Read the model definition and answer for the solid it produces. Units are mm, in the model's axes. Face numbers are marked on the shaded views. Give positions to 0.01 mm unless a question says otherwise; leave off trailing zeros. Loops run counter-clockwise (first coordinate to the right, second up) from the corner with the lowest first, then second, coordinate; pieces in that order, holes last. Notation, with made-up numbers: (-26, -37) - (29, -37) arc R23 cw to (29, 0) - close; hole circle Ø2 at (83, 16.5). An arc over 180 degrees is marked (long way). Write item = value, one per line.
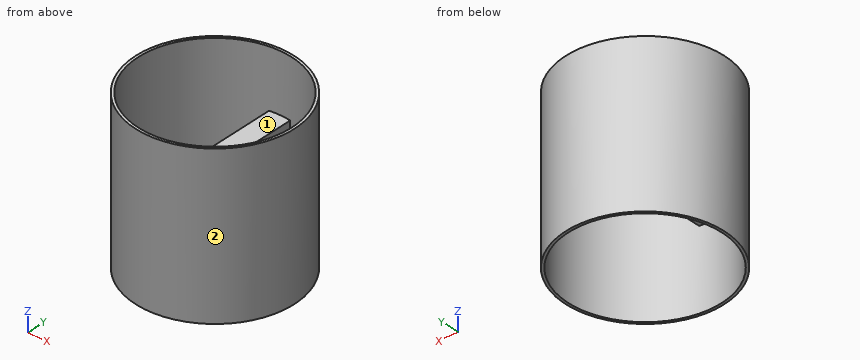
```python
from build123d import *

# Parameters (mm, degrees)
ESQUISSE1_W             = 8
ESQUISSE1_H             = 59
BOSS_EXTRU_1_DEPTH      = 60
ESQUISSE3_R             = 30
ESQUISSE3_R_2           = 29
BOSS_EXTRU_2_DEPTH      = 60
ESQUISSE4_R             = 29
ENL_V_MAT_EXTRU_3_DEPTH = 30
ENL_V_MAT_EXTRU_5_DEPTH = 1.5
ESQUISSE6_R             = 29
ENL_V_MAT_EXTRU_6_DEPTH = 22
ESQUISSE7_R             = 2
ENL_V_MAT_EXTRU_7_DEPTH = 6.5
ESQUISSE9_R             = 2
BOSS_EXTRU_4_DEPTH      = 6.5
ESQUISSE10_R            = 2
ENL_V_MAT_EXTRU_8_DEPTH = 3.7
ESQUISSE11_R            = 0.75
ENL_V_MAT_EXTRU_9_DEPTH = 3.7


with BuildPart() as part:
    # Esquisse1 → Boss.-Extru.1 (new body)
    with BuildSketch(Plane.XY):
        with Locations((4, 29.5)):
            Rectangle(ESQUISSE1_W, ESQUISSE1_H)
    extrude(amount=BOSS_EXTRU_1_DEPTH)

    # Esquisse3 → Boss.-Extru.2 (add)
    with BuildSketch(Plane(origin=(0, 0, 0), x_dir=(-1, 0, 0), z_dir=(0, 0, -1))):
        with Locations((-4, 29.5)):
            Circle(ESQUISSE3_R)
        with Locations((-4, 29.5)):
            Circle(ESQUISSE3_R_2, mode=Mode.SUBTRACT)
    extrude(amount=-BOSS_EXTRU_2_DEPTH)

    # Esquisse4 → Enlèv. mat.-Extru.3 (cut)
    with BuildSketch(Plane(origin=(0, 0, 0), x_dir=(-1, 0, 0), z_dir=(0, 0, -1))):
        with Locations((-4, 29.5)):
            Circle(ESQUISSE4_R)
    extrude(amount=-ENL_V_MAT_EXTRU_3_DEPTH, mode=Mode.SUBTRACT)

    # Esquisse5 → Enlèv. mat.-Extru.5 (cut)
    with BuildSketch(Plane(origin=(0, 0, 30), x_dir=(-1, 0, 0), z_dir=(0, 0, -1))):
        with BuildLine():
            Line((-6, 43), (-6.967257844, 29.9420191))
            ThreePointArc((-6.967257844, 29.9420191), (-7, 29.5), (-6.967257844, 29.0579809))
            Line((-6.967257844, 29.0579809), (-6, 16))
            ThreePointArc((-6, 16), (-4, 14), (-2, 16))
            Line((-2, 16), (-1.032742156, 29.0579809))
            ThreePointArc((-1.032742156, 29.0579809), (-1, 29.5), (-1.032742156, 29.9420191))
            Line((-1.032742156, 29.9420191), (-2, 43))
            ThreePointArc((-2, 43), (-4, 45), (-6, 43))
        make_face()
    extrude(amount=-ENL_V_MAT_EXTRU_5_DEPTH, mode=Mode.SUBTRACT)

    # Esquisse6 → Enlèv. mat.-Extru.6 (cut)
    with BuildSketch(Plane.XY.offset(60)):
        with Locations((4, 29.5)):
            Circle(ESQUISSE6_R)
    extrude(amount=-ENL_V_MAT_EXTRU_6_DEPTH, mode=Mode.SUBTRACT)

    # Esquisse7 → Enlèv. mat.-Extru.7 (cut)
    with BuildSketch(Plane(origin=(0, 0, 31.5), x_dir=(-1, 0, 0), z_dir=(0, 0, -1))):
        with Locations((-4, 29.5)):
            Circle(ESQUISSE7_R)
    extrude(amount=-ENL_V_MAT_EXTRU_7_DEPTH, mode=Mode.SUBTRACT)

    # Esquisse9 → Boss.-Extru.4 (add)
    with BuildSketch(Plane.XY.offset(38)):
        with Locations((4, 29.5)):
            Circle(ESQUISSE9_R)
    extrude(amount=-BOSS_EXTRU_4_DEPTH)

    # Esquisse10 → Enlèv. mat.-Extru.8 (cut)
    with BuildSketch(Plane.XY.offset(38)):
        with Locations((4, 29.5)):
            Circle(ESQUISSE10_R)
    extrude(amount=-ENL_V_MAT_EXTRU_8_DEPTH, mode=Mode.SUBTRACT)

    # Esquisse11 → Enlèv. mat.-Extru.9 (cut)
    with BuildSketch(Plane.XY.offset(34.3)):
        with Locations((4, 29.5)):
            Circle(ESQUISSE11_R)
    extrude(amount=-ENL_V_MAT_EXTRU_9_DEPTH, mode=Mode.SUBTRACT)


solid = part.part
```
1) A cutting plane is placed at C-C on z = 46. Determine the outline of the cut face in (x, y).
Output:
outline = circle Ø60 at (4, 29.5); hole circle Ø58 at (4, 29.5)
2) Find the intervals of material crossed by probe 1 along Y at (x, z) = (4, 36.05); probe 2 along Y at (x, z) = (4.5, 57.5); probe 3 along X at (y, z) = (43, 36), in increasing order.
Output:
probe_1 = -0.5 to 27.5, 31.5 to 59.5
probe_2 = -0.5 to 0.5, 58.5 to 59.5
probe_3 = -22.79 to -21.67, 0 to 8, 29.67 to 30.79
3) A cutting plane is placed at D-D on x = 17.5. Determine the outline of the cut face in (y, z).
Output:
outline = (2.71, 0) - (3.83, 0) - (3.83, 60) - (2.71, 60) - close; (55.17, 0) - (56.29, 0) - (56.29, 60) - (55.17, 60) - close
4) Each of these flat-tipped pins is pushed along its axis until it touches: P1, Ø4.5, axis at x = 4.5, y = 28.5, coming from the +Z side; P2, Ø1.5, axis at x = 9.5, y = 20, coming from the +Z side; P3, Ø4, axis at y = 41.5, z = 33.5, coming from the +X side; P4, Ø10, axis at x = -18.5, z = 12.5, coming from the -Y side. Where does it stop, or does it pass through?
Output:
P1 = 38
P2 = through
P3 = 32.28
P4 = 5.13
5) A cutting plane is placed at A-A on y = 11. Determine the outline of the cut face in (x, z), then the cut area to 3 significant figures.
Output:
outline = (-19.62, 0) - (-18.33, 0) - (-18.33, 60) - (-19.62, 60) - close; (0, 30) - (8, 30) - (8, 38) - (0, 38) - close; (26.33, 0) - (27.62, 0) - (27.62, 60) - (26.33, 60) - close
area = 218 mm²
6) The mould has two halves that part along Y. Classify the marked faces 1 and 2: pulls with the +Y half, pulls with the -Y half, needs draft (parallel to the pull), parting line crosses it, or undercut.
Output:
face_1 = undercut
face_2 = parting line crosses it
